Design review of the part built by this model. Coordinates are the model's own, in mm. A direction names the side the tool comes from. Coordinates: 2 decimals unless noted, no trailing zeros. Write each loop counter-clockwise with the first axis right and the second up, starting at its lowest first coordinate (ties: lowest second). Pieces come first, ordered by that corner, then holes. Notation, with made-up numbers: M 3.5,-19 L 32.5,-19 A27 ccw 32.5,0 Z; hole C -13.5,-29.5 d9. An arc over 180 degrees is marked long. Write item = value, one per line.
```python
from build123d import *

# Parameters (mm, degrees)
PAD003_DEPTH    = 1.3
SKETCH008_R     = 0.5
PAD004_DEPTH    = 0.8
SKETCH009_W     = 1.21537
SKETCH009_H     = 0.3
PAD005_DEPTH    = 3
CHAMFER001_SIZE = 0.3
CHAMFER002_SIZE = 0.3
CHAMFER003_SIZE = 0.2
CHAMFER004_SIZE = 0.4
SKETCH010_W     = 0.15
SKETCH010_H     = 0.4
PAD006_DEPTH    = 3.1


with BuildPart() as part:
    # Sketch007 → Pad003 (new body, symmetric)
    with BuildSketch(Plane.XY):
        Polygon((-2.75, 0), (2.75, 0), (2.75, 4.8), (1.5, 4.8), (1.5, 1.8), (-1.5, 1.8), (-1.5, 4.8), (-2.75, 4.8), align=None)
    extrude(amount=PAD003_DEPTH, both=True)

    # Sketch008 (on Face1 of Pad003) → Pad004 (join)
    with BuildSketch(Plane.XZ):
        with Locations((0, 0.75)):
            Circle(SKETCH008_R)
    extrude(amount=PAD004_DEPTH)

    # Sketch009 (on Face11 of Pad004) → Pad005 (join)
    with BuildSketch(Plane.YZ.offset(-1.5)):
        with Locations((4.05, 0)):
            Rectangle(SKETCH009_W, SKETCH009_H)
    extrude(amount=PAD005_DEPTH)

    # Chamfer001
    chamfer001_edges = [part.edges().sort_by_distance(p)[0] for p in [
        (-1.5, 1.8, 0),
        (1.5, 1.8, 0),
    ]]
    chamfer(chamfer001_edges, length=CHAMFER001_SIZE)

    # Chamfer002
    chamfer002_edges = [part.edges().sort_by_distance(p)[0] for p in [
        (-1.5, 3.45, 1.3),
        (-1.5, 3.45, -1.3),
        (1.5, 3.45, 1.3),
        (1.5, 3.45, -1.3),
    ]]
    chamfer(chamfer002_edges, length=CHAMFER002_SIZE)

    # Chamfer003
    chamfer003_edges = [part.edges().sort_by_distance(p)[0] for p in [
        (-0.5, -0.8, 0.75),
    ]]
    chamfer(chamfer003_edges, length=CHAMFER003_SIZE)

    # Chamfer004
    chamfer004_edges = [part.edges().sort_by_distance(p)[0] for p in [
        (2.275, 4.8, 1.3),
        (-2.275, 4.8, 1.3),
    ]]
    chamfer(chamfer004_edges, length=CHAMFER004_SIZE)

    # Sketch010 (on Face6 of Chamfer004) → Pad006 (join)
    with BuildSketch(Plane.XZ):
        with Locations((-2.275, 1)):
            Rectangle(SKETCH010_W, SKETCH010_H)
        with Locations((-2.275, -1)):
            Rectangle(SKETCH010_W, SKETCH010_H)
        with Locations((2.275, 1)):
            Rectangle(SKETCH010_W, SKETCH010_H)
        with Locations((2.275, -1)):
            Rectangle(SKETCH010_W, SKETCH010_H)
    extrude(amount=PAD006_DEPTH)


solid = part.part
```
Q1. Consider section C-C, the plane y = -1. State the section outline as (x, z) points, and give its area (3 significant figures).
Check result:
outline = M -2.35,-1.2 L -2.2,-1.2 L -2.2,-0.8 L -2.35,-0.8 Z; M -2.35,0.8 L -2.2,0.8 L -2.2,1.2 L -2.35,1.2 Z; M 2.2,-1.2 L 2.35,-1.2 L 2.35,-0.8 L 2.2,-0.8 Z; M 2.2,0.8 L 2.35,0.8 L 2.35,1.2 L 2.2,1.2 Z
area = 0.240 mm²
Q2. Consider section B-B, the plane x = 0. State the section outline as (y, z) points.
Check result:
outline = M -0.8,0.45 L -0.6,0.25 L 0,0.25 L 0,-1.3 L 1.8,-1.3 L 1.8,1.3 L 0,1.3 L 0,1.25 L -0.6,1.25 L -0.8,1.05 Z; M 3.44,-0.15 L 4.66,-0.15 L 4.66,0.15 L 3.44,0.15 Z
Q3. The part is to be moulded in two halves that separate along X. For faces 4 (the flat face through (0, 1, 1.3)), 5 (the flat face through (0, 4, -0.15)), 6 (the flat face through (2.75, 2, 0)), say which applies: +X half, -X half, draft (parallel to the pull), parting line (faces both ways), or undercut.
Check result:
face_4 = draft
face_5 = undercut
face_6 = +X half
Q4. Consider section D-D, the plane z = -0.4. State the section outline as (x, y) points, and give its area (3 significant figures).
Check result:
outline = M -2.75,0 L 2.75,0 L 2.75,4.8 L 1.5,4.8 L 1.5,2.1 L 1.2,1.8 L -1.2,1.8 L -1.5,2.1 L -1.5,4.8 L -2.75,4.8 Z
area = 17.5 mm²
Q5. Machinability: for faces 1 (the flat face through (-2, 4.8, 0)), 2 (the cylindrical face through (-0.108, -0.296, 0.262)), 3 (the flat face through (0, 4, 0.15)), which of the approach directions +Z, -Z, +X, -X, +Y, -Y give a long, thin tool a straight path to every point of the face, cutting with its end or side? Answer none if there is none.
Check result:
face_1 = +Z, -Z, +X, -X, +Y
face_2 = -Y
face_3 = +Z, +Y
Q6. For P1, Ø0.6, axis at x = 0, y = 4, coming from the -Z side; P2, Ø0.6, axis at x = 0.5, y = 4, coming from the +Z side; P3, Ø3, axis at x = -0.5, y = -2, coming from the +Z side, all flat-tipped, find the tip position at first contact; note any pin that passes through.
Check result:
P1 = -0.15
P2 = 0.15
P3 = 1.25
Q7. Consider section A-A, the plane y = 3.25. State the section outline as (x, z) points, and give its area (3 significant figures).
Check result:
outline = M -2.75,-1.3 L -1.8,-1.3 L -1.5,-1 L -1.5,1 L -1.8,1.3 L -2.75,1.3 Z; M 1.5,-1 L 1.8,-1.3 L 2.75,-1.3 L 2.75,1.3 L 1.8,1.3 L 1.5,1 Z
area = 6.32 mm²
Q8. Wall thickness on line 1 (X direction, y = 4, z = -0.95); line 2 (Y direction, x = 0.2, z = 0); line 3 (Y direction, x = 2.45, z = -0.9): over which ranges is each line inside the solid? List them lowest first.
Check result:
line_1 = -2.75 to -1.5, 1.5 to 2.75
line_2 = 0 to 1.8, 3.44 to 4.66
line_3 = 0 to 4.8
